The listing builds one solid part. Answer for the finished solid, in the listing's coordinates (mm). Face numbers are marked on the shaded views. A direction names the side the tool comes from. Give positions to 0.01 mm unless a question says otherwise; leave off trailing zeros. Order: outer loops, then holes, each group sorted by start corner. A loop starts at its lowest first (then second) coordinate and runs counter-clockwise, first axis right, second up. Notation, with made-up numbers: (-25, 84) - (1, 84) arc R16 ccw to (1, 97) - close; hole circle Ø3 at (43.5, -26.5). An arc over 180 degrees is marked (long way). Write each question's results on one line, items separated by ' | '. Start each with the question number.
1. Which of the six approach directions +Z, -Z, +X, -X, +Y, -Y give full straight-line access (tool end or side, diameter ignored) to the marked faces 4 and 5?
2. Section B-B (z = 2.5) is taken. Give the vertices of the cut face in (x, y), and give its area (3 significant figures).
3. Find the intervals of material crossed by L1, parallel to Y at x = 0, z = 1.95; L2, parallel to Y at x = 2.75, z = 1; L3, parallel to X at y = -1, z = 2.3, in increasing order.
4. Determine the mould class of the marked faces 1, 2 and 3 for opening direction X: released by +X, released by -X, zero draft, split by the parting line, or undercut.
5. Section D-D (y = 10.5) is taken. Give the vertices of the cut face in (x, z), and give its area (3 significant figures).
6. A flat-ended cylindrical pin translates along its axis: pin 1 (1.8 mm diameter, centred on y = 17.5, z = 1.5, fed in from +X). Find the tip coordinate at first contact, or state that the pin passes through.
7. Section C-C (y = 2.5) is taken. Give the vertices of the cut face in (x, z).
8. Section A-A (x = 0) is taken. Give the vertices of the cut face in (y, z), and give its area (3 significant figures).
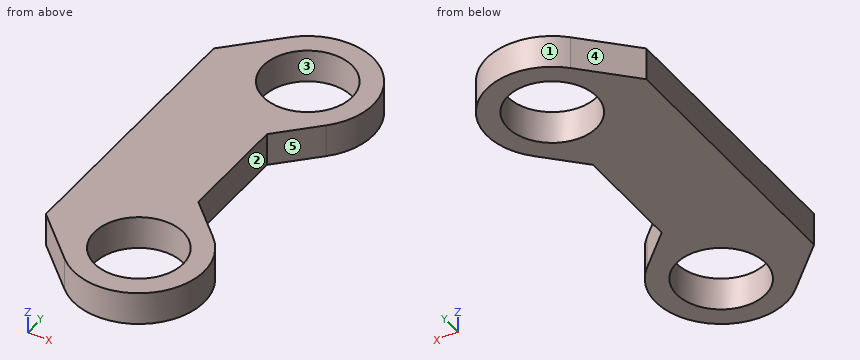
from build123d import *

# Parameters (mm, degrees)
CROQUIS1_R              = 7
CROQUIS1_R_2            = 4.75
SALIENTE_EXTRUIR1_DEPTH = 3.5
CROQUIS4_W              = 8.235883517
CROQUIS4_H              = 32.578937154
CORTAR_EXTRUIR4_DEPTH   = 4


with BuildPart() as part:
    # Croquis1 → Saliente-Extruir1 (new body)
    # profile 1 of 3: a face of its own
    with BuildSketch(Plane.XY):
        with BuildLine():
            ThreePointArc((-4.949747468, -4.949747468), (-4.949747468, 4.949747468), (4.949747468, 4.949747468))
            Line((4.949747468, 4.949747468), (1, 8.899494937))
            Line((1, 8.899494937), (1, 21.100505063))
            Line((1, 21.100505063), (4.949747468, 25.050252532))
            ThreePointArc((4.949747468, 25.050252532), (-4.949747468, 25.050252532), (-4.949747468, 34.949747468))
            Line((-4.949747468, 34.949747468), (-13, 26.899494937))
            Line((-13, 26.899494937), (-13, 3.100505063))
            Line((-13, 3.100505063), (-4.949747468, -4.949747468))
        make_face()
    # profile 2 of 3: a face of its own
    with BuildSketch(Plane.XY):
        with Locations((0, 30)):
            Circle(CROQUIS1_R)
        with Locations((0, 30)):
            Circle(CROQUIS1_R_2, mode=Mode.SUBTRACT)
    # profile 3 of 3: a face of its own
    with BuildSketch(Plane.XY):
        Circle(CROQUIS1_R)
        Circle(CROQUIS1_R_2, mode=Mode.SUBTRACT)
    extrude(amount=SALIENTE_EXTRUIR1_DEPTH)

    # Croquis4 → Cortar-Extruir4 (cut)
    with BuildSketch(Plane.XY.offset(3.5)):
        with Locations((-14.117941759, 13.61002636)):
            Rectangle(CROQUIS4_W, CROQUIS4_H)
    extrude(amount=-CORTAR_EXTRUIR4_DEPTH, mode=Mode.SUBTRACT)


solid = part.part
Reported:
1) face 4: +Z, -Z, -X, +Y | face 5: +Z, -Z, +X
2) outline: (-10, 0.1) - (-4.95, -4.95) arc R7 ccw to (4.95, 4.95) - (1, 8.9) - (1, 21.1) - (4.95, 25.05) arc R7 ccw to (-4.95, 34.95) - (-10, 29.9) - close; hole circle Ø9.5 at (0, 0); hole circle Ø9.5 at (0, 30) | area: 421 mm²
3) L1: -7 to -4.75, 4.75 to 25.25, 34.75 to 37 | L2: -6.44 to -3.87, 3.87 to 7.15, 22.85 to 26.13, 33.87 to 36.44 | L3: -8.9 to -4.64, 4.64 to 6.93
4) face 1: split by the parting line | face 2: released by +X | face 3: undercut
5) outline: (-10, 0) - (1, 0) - (1, 3.5) - (-10, 3.5) - close | area: 38.5 mm²
6) pin 1: x = 1
7) outline: (-10, 0) - (-4.04, 0) - (-4.04, 3.5) - (-10, 3.5) - close; (4.04, 0) - (6.54, 0) - (6.54, 3.5) - (4.04, 3.5) - close
8) outline: (-7, 0) - (-4.75, 0) - (-4.75, 3.5) - (-7, 3.5) - close; (4.75, 0) - (25.25, 0) - (25.25, 3.5) - (4.75, 3.5) - close; (34.75, 0) - (37, 0) - (37, 3.5) - (34.75, 3.5) - close | area: 87.5 mm²
